Geometry check sheet. Reference: the model listing, model coordinates, mm. A direction names the side the tool comes from. Give positions to 0.01 mm unless a question says otherwise; leave off trailing zeros. Loops run counter-clockwise (first coordinate to the right, second up) from the corner with the lowest first, then second, coordinate; pieces in that order, holes last. Notation, with made-up numbers: (16, 79) - (34, 79) arc R23 ccw to (34, 104) - close; hole circle Ø7 at (-35, 80). An arc over 180 degrees is marked (long way). Write item = value, one per line. Start each with the question number.
from build123d import *

# Parameters (mm, degrees)
BOSS_EXTRUDE1_DEPTH = 26
SKETCH2_R           = 4.5
BOSS_EXTRUDE2_DEPTH = 30
FILLET1_R           = 2
CHAMFER1_SIZE       = 5


with BuildPart() as part:
    # Sketch1 → Boss-Extrude1 (new body)
    with BuildSketch(Plane(origin=(0, 0, 0), x_dir=(1, 0, 0), z_dir=(0, 1, 0))):
        Polygon((-10, 0), (0, 0), (0, 20), (-30, 20), (-30, 15), (-5, 15), (-5, 5), (-10, 5), align=None)
        Polygon((0, 0), (10, 0), (10, 5), (5, 5), (5, 15), (30, 15), (30, 20), (0, 20), align=None)
    extrude(amount=BOSS_EXTRUDE1_DEPTH)

    # Sketch2 → Boss-Extrude2 (add)
    with BuildSketch(Plane.XY.offset(-15)):
        with Locations(Location((-25.5, 21.5, 0), (0, 0, 180))):
            Circle(SKETCH2_R)
    boss_extrude2 = extrude(amount=BOSS_EXTRUDE2_DEPTH)

    # Mirror1: Boss-Extrude2 across plane
    add(boss_extrude2.mirror(Plane(origin=(0, 0, 0), x_dir=(0, 0, 1), z_dir=(1, 0, 0))))

    # Fillet1
    fillet1_edges = [part.edges().sort_by_distance(p)[0] for p in [
        (-10, 13, 0),
        (10, 13, 0),
    ]]
    fillet(fillet1_edges, radius=FILLET1_R)

    # Chamfer1
    chamfer1_edges = [part.edges().sort_by_distance(p)[0] for p in [
        (5, 13, -5),
        (-5, 13, -5),
    ]]
    chamfer(chamfer1_edges, length=CHAMFER1_SIZE - 0.0001)  # a hair under: the kernel refuses the full size


solid = part.part
1) Material ranges on line 1 along X through (y, z) = (21.25, -7); line 2 along X through (y, z) = (22.5, -3); line 3 along Z through (x, y) = (0.5, 11.25), recorded low to high.
2) Gauge pin test, flat ends, axial feed: P1, Ø3, axis at y = 16.5, z = -6.5, coming from the +X side; P2, Ø2.5, axis at y = 11.5, z = -3.5, coming from the -X side; P3, Ø0.9, axis at y = 10.5, z = -4, coming from the +X side; P4, Ø4, axis at y = 12, z = -13.5, coming from the -X side. Record the tip position at first contact, or that the pin passes through.
3) Tool access check on faces 5 (the face through (-5, 13, -13)), 6 (the face through (-9.4, 13.18, -0.57)), 7 (the face through (22.18, 18.46, -0.21)), 8 (the face through (-29, 25, -15)). Record the directions out of +Z, -Z, +X, -X, +Y, -Y that give a thin tool (end or side, any length) a straight path to the whole face; none if there is none.
4) Cross-section at D-D on x = 17.5. Enter the section's corners in (y, z).
5) Cross-section at C-C on z = -1. Enter the section's corners in (x, y), and give its area (3 significant figures).
6) Release check for a two-part mould opening along Z. For faces 1 (the face through (0, 13, 0)), 2 (the face through (7, 13, -8)), 3 (the face through (5, 13, -12)), 4 (the face through (0, 0, -12)) record: pulls with the +Z half, pulls with the -Z half, needs draft (parallel to the pull), parting line crosses it, or undercut.
7) Cross-section at A-A on z = 11. Enter the section's corners in (x, y), and give its area (3 significant figures).
Checked values:
q1.line_1 = -29.99 to -21.01, -8 to 8, 21.01 to 29.99
q1.line_2 = -29.89 to -21.11, -10 to 10, 21.11 to 29.89
q1.line_3 = -20 to 0
q2.P1 = 28.33
q2.P2 = -10
q2.P3 = 10
q2.P4 = -30
q3.face_5 = +Y, -Y
q3.face_6 = +Z, +Y, -Y
q3.face_7 = +Z
q3.face_8 = +Z, -X, +Y
q4.outline = (0, -20) - (26, -20) - (26, -15) - (0, -15) - close
q5.outline = circle Ø9 at (-25.5, 21.5); (-9.73, 0) - (9.73, 0) - (9.73, 26) - (-9.73, 26) - close; circle Ø9 at (25.5, 21.5)
q5.area = 633 mm²
q6.face_1 = pulls with the +Z half
q6.face_2 = undercut
q6.face_3 = undercut
q6.face_4 = needs draft
q7.outline = circle Ø9 at (-25.5, 21.5); circle Ø9 at (25.5, 21.5)
q7.area = 127 mm²
